```python
from build123d import *

# Parameters (mm, degrees)
F0_R     = 1.5875
F0_R_2   = 12.3825
F1_DEPTH = 33.655
F2_W     = 6.016172
F2_H     = 2.024958
F3_DEPTH = 12.7
F4_R     = 12.3825
F4_R_2   = 1.5875
F5_DEPTH = 20.955


with BuildPart() as f1:
    # F0 (on Front) → F1 (new body)
    with BuildSketch(Plane.XZ):
        with BuildLine():
            ThreePointArc((40.760279, 16.387484), (36.015898, 13.31191), (40.802172, 10.301946))
            ThreePointArc((40.802172, 10.301946), (42.203223, 11.539621), (42.724182, 13.335))
            ThreePointArc((42.724182, 13.335), (42.190796, 15.14984), (40.760279, 16.387484))
        make_face()
        with Locations((39.37, 13.335)):
            Circle(F0_R, mode=Mode.SUBTRACT)
        with BuildLine():
            ThreePointArc((23.614713, 2.18623), (22.009207, 0.978353), (20.254373, 0))
            Line((20.254373, 0), (45.72, 0))
            Line((45.72, 0), (45.72, 26.67))
            Line((45.72, 26.67), (20.254373, 26.67))
            ThreePointArc((20.254373, 26.67), (22.360042, 25.45617), (24.237647, 23.912854))
            Line((24.237647, 23.912854), (40.760279, 16.387484))
            ThreePointArc((40.760279, 16.387484), (42.190796, 15.14984), (42.724182, 13.335))
            ThreePointArc((42.724182, 13.335), (42.203223, 11.539621), (40.802172, 10.301946))
            Line((40.802172, 10.301946), (23.614713, 2.18623))
        make_face()
        with BuildLine():
            ThreePointArc((0, 8.628126), (2.962228, 3.529669), (7.685627, 0))
            Line((7.685627, 0), (20.254373, 0))
            ThreePointArc((20.254373, 0), (22.009207, 0.978353), (23.614713, 2.18623))
            ThreePointArc((23.614713, 2.18623), (27.376982, 7.205693), (28.711627, 13.335))
            ThreePointArc((28.711627, 13.335), (27.547139, 19.077549), (24.237647, 23.912854))
            ThreePointArc((24.237647, 23.912854), (22.360042, 25.45617), (20.254373, 26.67))
            Line((20.254373, 26.67), (7.685627, 26.67))
            ThreePointArc((7.685627, 26.67), (2.962228, 23.140331), (0, 18.041874))
            Line((0, 18.041874), (0, 8.628126))
        make_face()
        with Locations((13.97, 13.335)):
            Circle(F0_R_2, mode=Mode.SUBTRACT)
        with BuildLine():
            Line((0, 26.67), (0, 18.041874))
            ThreePointArc((0, 18.041874), (2.962228, 23.140331), (7.685627, 26.67))
            Line((7.685627, 26.67), (0, 26.67))
        make_face()
        with BuildLine():
            Line((0, 8.628126), (0, 0))
            Line((0, 0), (7.685627, 0))
            ThreePointArc((7.685627, 0), (2.962228, 3.529669), (0, 8.628126))
        make_face()
        with BuildLine():
            ThreePointArc((28.711627, 13.335), (27.376982, 7.205693), (23.614713, 2.18623))
            Line((23.614713, 2.18623), (40.802172, 10.301946))
            ThreePointArc((40.802172, 10.301946), (36.015898, 13.31191), (40.760279, 16.387484))
            Line((40.760279, 16.387484), (24.237647, 23.912854))
            ThreePointArc((24.237647, 23.912854), (27.547139, 19.077549), (28.711627, 13.335))
        make_face()
    extrude(amount=-F1_DEPTH)

    # F2 (on face) → F3 (cut)
    with BuildSketch(Plane.XZ):
        with Locations((0, 13.335)):
            Rectangle(F2_W, F2_H)
    extrude(amount=-F3_DEPTH, mode=Mode.SUBTRACT)

    # F4 (on face) → F5 (join)
    with BuildSketch(Plane(origin=(0, 33.655, 0), x_dir=(-1, 0, 0), z_dir=(0, 1, 0))):
        with Locations((-13.97, 13.335)):
            Circle(F4_R)
        with Locations((-13.97, 13.335)):
            Circle(F4_R_2, mode=Mode.SUBTRACT)
    extrude(amount=-F5_DEPTH)


solid = f1.part
```
Build history of the part. All positions in model axes, mm. A direction names the side the tool comes from. Round coordinates to 2 decimals unless told otherwise and drop trailing zeros. Write each loop counter-clockwise with the first axis right and the second up, starting at its lowest first coordinate (ties: lowest second). Pieces come first, ordered by that corner, then holes. Notation, with made-up numbers: (23.5, 39.5) - (50.5, 39.5) arc R19 cw to (50.5, 71.5) - close; hole circle Ø7 at (61.5, -20). An arc over 180 degrees is marked (long way). Write each question's results on one line, items separated by ' | '. Start each with the question number.
Item 1: Mould opens along X. For faces 4 (the face through (45.72, 17, 13)), 5 (the face through (15.23, 23.32, 12.37)), 6 (the face through (1, 6, 14.347)), 7 (the face through (0, 17, 14)) say: pulls with the +X half, pulls with the -X half, needs draft (parallel to the pull), parting line crosses it, or undercut.
Item 2: Drop flat-ended pins along their axis: P1, Ø1.9, axis at x = 13.97, z = 13.335, coming from the +Y side; P2, Ø7.5, axis at x = 14.5, z = 9, coming from the -Y side. Give the stop position or say it passes through.
Item 3: Saw through at B-B (y = 9.5). Write the cut outline in (x, z) (1 decimal), and give its area (3 significant figures).
Item 4: Saw through at C-C (z = 5.5). Write the cut outline in (x, y) (3 decimals), and give its area (3 significant figures).
Item 5: Saw through at A-A (x = 13.97). Write the cut outline in (y, z) (1 decimal), and give its area (3 significant figures).
Item 6: Saw through at D-D (x = 39.37). Write the cut outline in (y, z) (1 decimal).
Item 7: Wall check: L1, parallel to Z at x = 13.97, y = 18; L2, parallel to X at y = 14, z = 14; L3, parallel to X at y = 24.5, z = 14.75. Give the ranges that are in metal, low to high. Write a range as [from, to].
Item 8: Which spindle directions (+Z, -Z, +X, -X, +Y, -Y) get a long thin tool onto all of the face, cutting with end or side? Do faces 1 (the face through (1, 6, 12.323)), 2 (the face through (16, 12.7, 14)), 3 (the face through (23, 17, 0)). Say none if no direction does.
Results are:
1) face 4: pulls with the +X half | face 5: undercut | face 6: needs draft | face 7: pulls with the -X half
2) P1: passes through | P2: stops at y = 12.7
3) outline: (0, 0) - (45.7, 0) - (45.7, 26.7) - (0, 26.7) - (0, 14.3) - (1.6, 14.3) arc R12.4 cw (long way) to (1.6, 12.3) - (0, 12.3) - close; hole circle Ø3.2 at (39.4, 13.3) | area: 727 mm²
4) outline: (0, 0) - (4.382, 0) - (4.382, 12.7) - (23.558, 12.7) - (23.558, 0) - (45.72, 0) - (45.72, 33.655) - (0, 33.655) - close | area: 1,300 mm²
5) outline: (0, 0) - (33.7, 0) - (33.7, 11.7) - (12.7, 11.7) - (12.7, 1) - (0, 1) - close; (0, 25.7) - (12.7, 25.7) - (12.7, 14.9) - (33.7, 14.9) - (33.7, 26.7) - (0, 26.7) - close | area: 517 mm²
6) outline: (0, 0) - (33.7, 0) - (33.7, 11.7) - (0, 11.7) - close; (0, 14.9) - (33.7, 14.9) - (33.7, 26.7) - (0, 26.7) - close
7) L1: z = [0, 11.75], [14.92, 26.67] | L2: x = [0, 12.53], [15.41, 37.93], [40.81, 45.72] | L3: x = [0, 13.25], [14.69, 38.65], [40.09, 45.72]
8) face 1: -X, -Y | face 2: -Y | face 3: -Z, +X, -X, +Y, -Y
